```python
from build123d import *

# Parameters (mm, degrees)
F1_DEPTH = 57.15
F3_DEPTH = 25.4


with BuildPart() as f1:
    # F0 (on Top) → F1 (new body)
    with BuildSketch(Plane.XY):
        Polygon((0.051027, -7.332171), (6.37536, -3.621895), (6.324333, 3.710276), (-0.051027, 7.332171), (-6.37536, 3.621895), (-6.324333, -3.710276), align=None)
    extrude(amount=F1_DEPTH)

    # F2 (on Top) → F3 (join)
    with BuildSketch(Plane.XY):
        with BuildLine():
            Line((-2.073388, -2.404514), (2.073388, -2.404514))
            ThreePointArc((2.073388, -2.404514), (0, 3.175), (-2.073388, -2.404514))
        make_face()
    extrude(amount=-F3_DEPTH)


solid = f1.part
```
Part model, mm, in its own coordinate system. A direction names the side the tool comes from. Round coordinates to 2 decimals unless told otherwise and drop trailing zeros. Loops run counter-clockwise (first coordinate to the right, second up) from the corner with the lowest first, then second, coordinate; pieces in that order, holes last.
Item 1: Cut at C-C, the plane x = -1.25. Give the cut face in (y, z).
Item 2: Cut at B-B, the plane z = 52. Give the cut face in (x, y).
Item 3: Drill centre lines: line 1 (Z direction, x = 6, y = 2); line 2 (X direction, y = -2.5, z = 13.5); line 3 (Y direction, x = -1.75, z = 33). Where is each one in solid material? Low to high.
Item 4: Drop flat-ended pins along their axis: P1, Ø4, axis at x = -4.5, z = 0, coming from the -Y side; P2, Ø6, axis at x = -1, y = -3, coming from the -Z side; P3, Ø2, axis at x = 1, z = -14.5, coming from the -Y side. Give the stop position or say it passes through.
Item 5: Cut at A-A, the plane y = 0. Give the cut face in (x, z) (3 decimals).
Item 6: 3-axis set-ups, long thin cutter, end or side, ignore diameter. For faces 1 (the face through (0, -2.405, -13)), 2 (the face through (0.108, 3.173, -12.522)), 3 (the face through (3.169, -5.503, 28.175)): which of +Z, -Z, +X, -X, +Y, -Y reach the whole face in a straight line?
Item 7: Cut at D-D, the plane z = -18.5. Give the cut face in (x, y) (3 decimals).
A:
1. outline: (-6.59, 0) - (-2.4, 0) - (-2.4, -25.4) - (2.92, -25.4) - (2.92, 0) - (6.63, 0) - (6.63, 57.15) - (-6.59, 57.15) - close
2. outline: (-6.38, 3.62) - (-6.32, -3.71) - (0.05, -7.33) - (6.38, -3.62) - (6.32, 3.71) - (-0.05, 7.33) - close
3. line 1: z = 0 to 57.15
3. line 2: x = -6.33 to 6.37
3. line 3: y = -6.31 to 6.34
4. P1: stops at y = -5.88
4. P2: stops at z = -25.4
4. P3: stops at y = -2.4
5. outline: (-6.35, 0) - (-3.175, 0) - (-3.175, -25.4) - (3.175, -25.4) - (3.175, 0) - (6.35, 0) - (6.35, 57.15) - (-6.35, 57.15) - close
6. face 1: -Z, +X, -X, -Y
6. face 2: -Z
6. face 3: +Z, -Z, +X, -Y
7. outline: (-2.073, -2.405) - (2.073, -2.405) arc R3.175 ccw (long way) to start
